```python
from build123d import *

# Parameters (mm, degrees)
F0_R     = 3.175
F1_DEPTH = 3.048


with BuildPart() as f1:
    # F0 (on Front) → F1 (new body)
    with BuildSketch(Plane.XZ):
        with BuildLine():
            ThreePointArc((-9.4502929642, 116.4222056828), (-0.596483242, 105.7252757886), (9.525, 115.2315806828))
            ThreePointArc((9.525, 115.2315806828), (9.5063048942, 115.8280639248), (9.4502929642, 116.4222056828))
            ThreePointArc((9.4502929642, 116.4222056828), (0, 124.7565806828), (-9.4502929642, 116.4222056828))
        make_face()
        with Locations((0, 115.2315806828)):
            Circle(F0_R, mode=Mode.SUBTRACT)
        with BuildLine():
            ThreePointArc((9.4502929642, 116.4222056828), (9.5063048942, 115.8280639248), (9.525, 115.2315806828))
            ThreePointArc((9.525, 115.2315806828), (-0.596483242, 105.7252757886), (-9.4502929642, 116.4222056828))
            Line((-9.4502929642, 116.4222056828), (-15.7504882737, 66.4159556828))
            ThreePointArc((-15.7504882737, 66.4159556828), (0, 80.3065806828), (15.7504882737, 66.4159556828))
            Line((15.7504882737, 66.4159556828), (9.4502929642, 116.4222056828))
        make_face()
        with Locations((-3.175, 100.9567806828)):
            Circle(F0_R, mode=Mode.SUBTRACT)
        with BuildLine():
            ThreePointArc((15.875, 64.4315806828), (15.8438414904, 65.4257194194), (15.7504882737, 66.4159556828))
            ThreePointArc((15.7504882737, 66.4159556828), (0, 80.3065806828), (-15.7504882737, 66.4159556828))
            ThreePointArc((-15.7504882737, 66.4159556828), (-15.8735137675, 64.6488033167), (-15.7988908218, 62.8789462115))
            ThreePointArc((-15.7988908218, 62.8789462115), (-0.0350334036, 48.5566193392), (15.7918841581, 62.8092306167))
            ThreePointArc((15.7918841581, 62.8092306167), (15.8542074228, 63.6193418048), (15.875, 64.4315806828))
        make_face()
        with Locations((0, 64.4315806828)):
            Circle(F0_R, mode=Mode.SUBTRACT)
        with BuildLine():
            ThreePointArc((15.7918841581, 62.8092306167), (-0.0350334036, 48.5566193392), (-15.7988908218, 62.8789462115))
            Line((-15.7988908218, 62.8789462115), (-9.6194684488, 0))
            ThreePointArc((-9.6194684488, 0), (-0.6064835851, 10.4451574562), (9.3848660442, 0.9315806828))
            ThreePointArc((9.3848660442, 0.9315806828), (6.6444220698, -5.7538829911), (0, -8.5923884202))
            Line((0, -8.5923884202), (44.566778303, -7.9366409191))
            ThreePointArc((44.566778303, -7.9366409191), (36.5142317093, 0.1657947093), (44.898157601, 7.9248382327))
            Line((44.898157601, 7.9248382327), (18.664461469, 9.408380228))
            ThreePointArc((18.664461469, 9.408380228), (13.0633502744, 12.1880545359), (11.2047605357, 18.158371115))
            Line((11.2047605357, 18.158371115), (12.2217881669, 28.0580733262))
            Line((12.2217881669, 28.0580733262), (9.806785479, 28.0580733262))
            Line((9.806785479, 28.0580733262), (9.806785479, 28.294084817))
            Line((9.806785479, 28.294084817), (10.6072340892, 28.4135123184))
            Line((10.6072340892, 28.4135123184), (10.0157836063, 30.1324152843))
            Line((10.0157836063, 30.1324152843), (7.6698862582, 30.1324152843))
            Line((7.6698862582, 30.1324152843), (7.0699052395, 28.4135123184))
            Line((7.0699052395, 28.4135123184), (7.8703538498, 28.294084817))
            Line((7.8703538498, 28.294084817), (7.8703538498, 28.0580733262))
            Line((7.8703538498, 28.0580733262), (5.9111741252, 28.0580733262))
            Line((5.9111741252, 28.0580733262), (5.9111741252, 28.294084817))
            Line((5.9111741252, 28.294084817), (6.5865082102, 28.4135123184))
            Line((6.5865082102, 28.4135123184), (8.6167757333, 34.0649922933))
            Line((8.6167757333, 34.0649922933), (9.4598770226, 34.0649922933))
            Line((9.4598770226, 34.0649922933), (11.5711846359, 28.4135123184))
            Line((11.5711846359, 28.4135123184), (12.2473153484, 28.3065537876))
            Line((12.2473153484, 28.3065537876), (15.7918841581, 62.8092306167))
        make_face()
        Polygon((-7.8443148705, 34.0166525904), (-5.9078832413, 34.0166525904), (-5.9078832413, 33.7806410996), (-6.5604692309, 33.6654788662), (-8.9561280379, 27.9201629973), (-9.1821872369, 27.9201629973), (-11.6034376513, 33.6654788662), (-12.2745064684, 33.7806410996), (-12.2745064684, 34.0166525904), (-9.8660518577, 34.0166525904), (-9.8660518577, 33.7806410996), (-10.666500468, 33.6654788662), (-8.862292144, 29.2793617032), (-7.0623490878, 33.6654788662), (-7.8443148705, 33.7806410996), align=None, mode=Mode.SUBTRACT)
        with BuildLine():
            Line((-5.5439137134, 28.0580733262), (-5.5439137134, 28.294084817))
            Line((-5.5439137134, 28.294084817), (-4.7790090023, 28.4135123184))
            Line((-4.7790090023, 28.4135123184), (-4.7790090023, 33.6654788662))
            Line((-4.7790090023, 33.6654788662), (-5.5439137134, 33.7806410996))
            Line((-5.5439137134, 33.7806410996), (-5.5439137134, 34.0166525904))
            Line((-5.5439137134, 34.0166525904), (-1.0739129483, 34.0166525904))
            Line((-1.0739129483, 34.0166525904), (-1.0739129483, 32.5906313539))
            Line((-1.0739129483, 32.5906313539), (-1.3667946778, 32.5906313539))
            Line((-1.3667946778, 32.5906313539), (-1.5089702747, 33.5545819006))
            add(Edge.make_bspline(
                [(-1.5089702747, 33.5545819006), (-2.0065848637, 33.6157174073), (-2.9492090708, 33.6157174073)],
                knots=[0, 0, 0, 1, 1, 1], degree=2))
            Line((-2.9492090708, 33.6157174073), (-3.9216901533, 33.6157174073))
            Line((-3.9216901533, 33.6157174073), (-3.9216901533, 31.2883028868))
            Line((-3.9216901533, 31.2883028868), (-2.3136841529, 31.2883028868))
            Line((-2.3136841529, 31.2883028868), (-2.1757738239, 31.999180871))
            Line((-2.1757738239, 31.999180871), (-1.8914226302, 31.999180871))
            Line((-1.8914226302, 31.999180871), (-1.8914226302, 30.1679591835))
            Line((-1.8914226302, 30.1679591835), (-2.1757738239, 30.1679591835))
            Line((-2.1757738239, 30.1679591835), (-2.3136841529, 30.8887894596))
            Line((-2.3136841529, 30.8887894596), (-3.9216901533, 30.8887894596))
            Line((-3.9216901533, 30.8887894596), (-3.9216901533, 28.4575867534))
            Line((-3.9216901533, 28.4575867534), (-2.7487414792, 28.4575867534))
            add(Edge.make_bspline(
                [(-2.7487414792, 28.4575867534), (-1.6028061686, 28.4575867534), (-1.2473671765, 28.5286745518)],
                knots=[0, 0, 0, 1, 1, 1], degree=2))
            Line((-1.2473671765, 28.5286745518), (-0.9942946141, 29.6305354274))
            Line((-0.9942946141, 29.6305354274), (-0.6999911286, 29.6305354274))
            Line((-0.6999911286, 29.6305354274), (-0.7852964867, 28.0580733262))
            Line((-0.7852964867, 28.0580733262), (-5.5439137134, 28.0580733262))
        make_face(mode=Mode.SUBTRACT)
        with BuildLine():
            Line((2.7065361721, 30.6712607964), (1.6359539277, 30.6712607964))
            Line((1.6359539277, 30.6712607964), (1.6359539277, 28.4135123184))
            Line((1.6359539277, 28.4135123184), (2.5373472118, 28.294084817))
            Line((2.5373472118, 28.294084817), (2.5373472118, 28.0580733262))
            Line((2.5373472118, 28.0580733262), (0.0720223624, 28.0580733262))
            Line((0.0720223624, 28.0580733262), (0.0720223624, 28.294084817))
            Line((0.0720223624, 28.294084817), (0.7786350787, 28.4135123184))
            Line((0.7786350787, 28.4135123184), (0.7786350787, 33.6654788662))
            Line((0.7786350787, 33.6654788662), (0.0137303676, 33.7806410996))
            Line((0.0137303676, 33.7806410996), (0.0137303676, 34.0166525904))
            Line((0.0137303676, 34.0166525904), (2.5871086707, 34.0166525904))
            add(Edge.make_bspline(
                [(2.5871086707, 34.0166525904), (3.7060306179, 34.0166525904), (4.2391891061, 33.6384655028)],
                knots=[0, 0, 0, 1, 1, 1], degree=2))
            add(Edge.make_bspline(
                [(4.2391891061, 33.6384655028), (4.7723475943, 33.2602784151), (4.7723475943, 32.4257076616)],
                knots=[0, 0, 0, 1, 1, 1], degree=2))
            add(Edge.make_bspline(
                [(4.7723475943, 32.4257076616), (4.7723475943, 31.8299919108), (4.4481872335, 31.3970672184)],
                knots=[0, 0, 0, 1, 1, 1], degree=2))
            add(Edge.make_bspline(
                [(4.4481872335, 31.3970672184), (4.1240268727, 30.9641425259), (3.5510592174, 30.7949535657)],
                knots=[0, 0, 0, 1, 1, 1], degree=2))
            Line((3.5510592174, 30.7949535657), (5.1633304857, 28.4135123184))
            Line((5.1633304857, 28.4135123184), (5.8073859394, 28.294084817))
            Line((5.8073859394, 28.294084817), (5.8073859394, 28.0580733262))
            Line((5.8073859394, 28.0580733262), (4.381364703, 28.0580733262))
            Line((4.381364703, 28.0580733262), (2.7065361721, 30.6712607964))
        make_face(mode=Mode.SUBTRACT)
        with BuildLine():
            ThreePointArc((9.3848660442, 0.9315806828), (-0.6064835851, 10.4451574562), (-9.6194684488, 0))
            ThreePointArc((-9.6194684488, 0), (-6.4854039547, -6.1721629528), (0, -8.5923884202))
            ThreePointArc((0, -8.5923884202), (6.6444220698, -5.7538829911), (9.3848660442, 0.9315806828))
        make_face()
        Circle(F0_R, mode=Mode.SUBTRACT)
        Polygon((12.3261370552, 28.294084817), (12.2473153484, 28.3065537876), (12.2217881669, 28.0580733262), (12.3261370552, 28.0580733262), align=None)
        Polygon((12.2217881669, 28.0580733262), (12.2473153484, 28.3065537876), (11.5711846359, 28.4135123184), (9.4598770226, 34.0649922933), (8.6167757333, 34.0649922933), (6.5865082102, 28.4135123184), (5.9111741252, 28.294084817), (5.9111741252, 28.0580733262), (7.8703538498, 28.0580733262), (7.8703538498, 28.294084817), (7.0699052395, 28.4135123184), (7.6698862582, 30.1324152843), (10.0157836063, 30.1324152843), (10.6072340892, 28.4135123184), (9.806785479, 28.294084817), (9.806785479, 28.0580733262), align=None)
        Polygon((7.8035313193, 30.5333504675), (8.8257738607, 33.4252021075), (9.8778732774, 30.5333504675), align=None, mode=Mode.SUBTRACT)
        with BuildLine():
            ThreePointArc((44.898157601, 7.9248382327), (36.5142317093, 0.1657947093), (44.566778303, -7.9366409191))
            ThreePointArc((44.566778303, -7.9366409191), (50.1037966903, -5.571219726), (52.3875, 0))
            ThreePointArc((52.3875, 0), (50.2189321892, 5.4519104584), (44.898157601, 7.9248382327))
        make_face()
        with Locations((44.45, 0)):
            Circle(F0_R, mode=Mode.SUBTRACT)
    extrude(amount=F1_DEPTH)


solid = f1.part
```
Could you check a few things on this model? Use its own coordinates, in mm. A direction names the side the tool comes from. Round coordinates to 2 decimals unless told otherwise and drop trailing zeros. Loops run counter-clockwise (first coordinate to the right, second up) from the corner with the lowest first, then second, coordinate; pieces in that order, holes last. Notation, with made-up numbers: M -28,60.5 L -18,60.5 A25 cw -18,74.5 Z; hole C -20,72 d7. An arc over 180 degrees is marked long. Write item = value, one per line.
1. I need wall thicknesses on probe 1 along Z at (x, y) = (44.45, -2.1) (3 decimals); probe 2 along Z at (x, y) = (2.5, -2.85); probe 3 along Z at (x, y) = (-6, -0.35). Which ranges of each line are inside material? Lowest first, please.
Results below:
probe_1 = -7.938 to -3.175, 3.175 to 7.95
probe_2 = -8.56 to -1.96, 1.96 to 28.06, 28.3 to 30.67, 34.02 to 62.47, 66.39 to 113.27, 117.19 to 124.42
probe_3 = -6.58 to 33.76, 34.02 to 99.51, 102.41 to 122.63
2. I want a section at B-B, the plane x = 28. Write out the boundary of the cut face in (y, z), and give its area (3 significant figures).
Results below:
outline = M -3.05,-8.18 L 0,-8.18 L 0,8.88 L -3.05,8.88 Z
area = 52.0 mm²
3. I want a section at A-A, the plane z = 53. Write out the boundary of the cut face in (x, y), and give its area (3 significant figures).
Results below:
outline = M -14.83,-3.05 L 14.78,-3.05 L 14.78,0 L -14.83,0 Z
area = 90.3 mm²
4. Will these pins go through, and if not, where does the flat tip stop? P1, Ø1.5, axis at y = -1.5, z = 31, coming from the -X side; P2, Ø1.2, axis at y = -2, z = 29.5, coming from the -X side.
Results below:
P1 = -12.74
P2 = -12.58
5. Which directions (+Z, -Z, +X, -X, +Y, -Y) give clear straight access to the entire face, cutting with the end or side of a thin tool? Please do faces 1 (the face through (1.636, -2, 30)), 2 (the face through (31.965, -1.503, 8.656)).
Results below:
face_1 = +Y, -Y
face_2 = +Z, +X, +Y, -Y
6. Thinking about a two-plate mould opening in X: for faces 3 (the face through (41.28, -1.5, 0.14)), 4 (the face through (-12.556, -1.503, 91.769)), 5 (the face through (-7.975, -1.503, 31.442)), 6 (the face through (12.644, -1.503, 91.069)), which applies, +X half, -X half, draft (parallel to the pull), parting line (faces both ways), or undercut?
Results below:
face_3 = undercut
face_4 = -X half
face_5 = undercut
face_6 = +X half
